The listing builds one solid part. Answer for the finished solid, in the listing's coordinates (mm). A direction names the side the tool comes from. Round coordinates to 2 decimals unless told otherwise and drop trailing zeros. Write each loop counter-clockwise with the first axis right and the second up, starting at its lowest first coordinate (ties: lowest second). Pieces come first, ordered by that corner, then holes. Notation, with made-up numbers: (-26, -25) - (27, -25) arc R34 cw to (27, 6) - close; hole circle Ø3 at (47, 44.25). An arc over 180 degrees is marked (long way). Answer as CSV lines item,"result". Start each with the question number.
Item 1: A cutting plane is placed at C-C on y = 0. Determine the outline of the cut face in (x, z) (3 decimals), and give its area (3 significant figures).
Item 2: Flat-ended cylindrical pins translate along their axes: pin 1 (5 mm diameter, centred on x = 14, z = 330, fed in from -Y); pin 2 (4 mm diameter, centred on y = 22, z = 83, fed in from +X); pin 3 (4 mm diameter, centred on x = -6.5, z = 333.5, fed in from +Y). Find the tip coordinate at first contact, or state that the pin passes through.
Item 3: A cutting plane is placed at B-B on z = 319.5. Determine the outline of the cut face in (x, y), and give its area (3 significant figures).
Item 4: Which of the six approach directions +Z, -Z, +X, -X, +Y, -Y give full straight-line access (tool end or side, diameter ignored) to faces 5 (the flat face through (12.7, -37, 9)), 6 (the flat face through (0, -50.8, 9)), 7 (the cylindrical face through (-0.931, 25.383, 9.392)), 8 (the cylindrical face through (-6.883, 30.995, 188.1))?
Item 5: A cutting plane is placed at D-D on y = -42. Determine the outline of the cut face in (x, z), and give its area (3 significant figures).
Item 6: A cutting plane is placed at A-A on x = 0. Determine the outline of the cut face in (y, z) (3 decimals).
Item 7: For a pull along Z with two mould halves and no side action, classify faces 1 (the flat face through (0, 0, -6.35)), 2 (the cylindrical face through (-2.507, -25.728, 374.647)), 3 (the flat face through (-12.7, -37, 9)), 4 (the flat face through (0, 0, 381)) as pulls with the +Z half, pulls with the -Z half, needs draft (parallel to the pull), parting line crosses it, or undercut.
Item 8: Straight lines are drawn through the part: line 1 along Z through (x, y) = (-21, 13); line 2 along X through (y, z) = (19, 46); line 3 along Z through (x, y) = (5.5, -45). For each, find the intervals that lie inside material, in ascending order. Write a range as [from, to].
Solid Edge part; units mm, degrees
sketch "Sketch1" plane through (0, 0, 0) normal (0, 0, 1) x (1, 0, 0)
  line L0 (12.7, -50.8) -> (12.7, -21.997)
  line L1 (0, -50.8) -> (12.7, -50.8)
  line L2 (0, -50.8) -> (-12.7, -50.8)
  line L3 (-12.7, -50.8) -> (-12.7, -21.997)
  arc A0 (-12.7, -21.997) -> (12.7, -21.997) centre (0, 0) cw
extrude "Protrusion1" add sketch "Sketch1" along normal blind 19.05
sketch "Sketch2" plane through (0, -12.7, 0) normal (0, 0, -1) x (0, -1, 0)
  circle A0 centre (-12.7, 0) radius 34.925
extrude "ExtrudedProtrusion_2" add sketch "Sketch2" along normal blind 6.35
fillet "Round_1" radius 12.7 1 edges at (0, 34.925, -6.35)
sketch "Sketch3" plane through (0, -12.7, 19.05) normal (0, 0, 1) x (1, 0, 0)
  circle A0 centre (0, 12.7) radius 31.75
extrude "ExtrudedProtrusion_3" add sketch "Sketch3" along normal blind 342.9
sketch "Sketch4" plane through (0, 0, 361.95) normal (0, 0, 1) x (1, 0, 0)
  circle A0 centre (0, 0) radius 25.4
extrude "ExtrudedProtrusion_4" add sketch "Sketch4" along normal blind 19.05
sketch "Sketch5" plane through (0, 0, 374.65) normal (0, 0, 1) x (1, 0, 0)
  circle A0 centre (0, 0) radius 31.75
extrude "ExtrudedProtrusion_5" add sketch "Sketch5" along normal blind 6.35 and the other way blind 1.27
sketch "Sketch6" plane through (0, 0, 374.65) normal (0, -1, 0) x (-1, 0, 0)
  line L0 (-63.5, 1.8054) -> (63.5, 1.8054)
  arc A0 (-63.5, 1.8054) -> (63.5, 1.8054) centre (0, 1117.6) ccw
extrude "Cutout1" cut sketch "Sketch6" along normal through all and the other way through all
sketch "Sketch7" plane through (0, 0, 361.95) normal (0, 0, 1) x (1, 0, 0)
  circle A0 centre (0, 0) radius 25.4
extrude "Protrusion2" add sketch "Sketch7" along normal up to vertex (19.05 mm away)
Geometry says:
1,outline,"(-34.925, 0) arc R12.7 ccw to (-23.926, -6.35) - (23.926, -6.35) arc R12.7 ccw to (34.925, 0) - (25.4, 0) - (25.4, 19.05) - (31.75, 19.05) - (31.75, 361.95) - (25.4, 361.95) - (25.4, 374.361) arc R1117.6 cw to (31.75, 374.199) - (31.75, 381) - (-31.75, 381) - (-31.75, 374.199) arc R1117.6 cw to (-25.4, 374.361) - (-25.4, 361.95) - (-31.75, 361.95) - (-31.75, 19.05) - (-25.4, 19.05) - (-25.4, 0) - close"
1,area,"24,200 mm^2"
2,pin 1,"stops at y = -29.59"
2,pin 2,"stops at x = 24.66"
2,pin 3,"stops at y = 31.43"
3,outline,"circle Ø63.5 at (0, 0)"
3,area,"3,170 mm^2"
4,face 5,"+X, -Y"
4,face 6,"+Z, -Z, +X, -X, -Y"
4,face 7,"none"
4,face 8,"+Z"
5,outline,"(-12.7, 0) - (12.7, 0) - (12.7, 19.05) - (-12.7, 19.05) - close"
5,area,"484 mm^2"
6,outline,"(-50.8, 0) - (-34.925, 0) arc R12.7 ccw to (-23.926, -6.35) - (23.926, -6.35) arc R12.7 ccw to (34.925, 0) - (25.4, 0) - (25.4, 19.05) - (31.75, 19.05) - (31.75, 361.95) - (25.4, 361.95) - (25.4, 374.65) - (31.75, 374.65) - (31.75, 381) - (-31.75, 381) - (-31.75, 374.65) - (-25.4, 374.65) - (-25.4, 361.95) - (-31.75, 361.95) - (-31.75, 19.05) - (-50.8, 19.05) - close"
7,face 1,"pulls with the -Z half"
7,face 2,"undercut"
7,face 3,"undercut"
7,face 4,"pulls with the +Z half"
8,line 1,"z = [-6.33, 381]"
8,line 2,"x = [-25.44, 25.44]"
8,line 3,"z = [0, 19.05]"
